```python
from build123d import *

# Parameters (mm, degrees)
SKETCH1_R                = 0.45
BOSS_EXTRUDE1_DEPTH      = 1
SKETCH2_R                = 0.75
BOSS_EXTRUDE2_DEPTH      = 0.5
SKETCH3_R                = 0.125
BOSS_EXTRUDE3_DEPTH      = 4
BOSS_EXTRUDE3_DEPTH_BACK = 20
CHAMFER1_SIZE            = 0.1


with BuildPart() as part:
    # Sketch1 → Boss-Extrude1 (new body)
    with BuildSketch(Plane(origin=(0, 0, 0), x_dir=(1, 0, 0), z_dir=(0, 1, 0))):
        Circle(SKETCH1_R)
    extrude(amount=BOSS_EXTRUDE1_DEPTH)

    # Sketch2 → Boss-Extrude2 (add)
    with BuildSketch(Plane(origin=(0, 1, 0), x_dir=(1, 0, 0), z_dir=(0, 1, 0))):
        Circle(SKETCH2_R)
    extrude(amount=BOSS_EXTRUDE2_DEPTH)

    # Sketch3 → Boss-Extrude3 (add, two sides)
    with BuildSketch(Plane.XY) as boss_extrude3_sk:
        with Locations((0, 1.25)):
            Circle(SKETCH3_R)
    extrude(amount=BOSS_EXTRUDE3_DEPTH)
    extrude(boss_extrude3_sk.sketch, amount=-BOSS_EXTRUDE3_DEPTH_BACK)

    # Chamfer1
    chamfer1_edges = [part.edges().sort_by_distance(p)[0] for p in [
        (-0.75, 1.5, 0),
    ]]
    chamfer(chamfer1_edges, length=CHAMFER1_SIZE)


solid = part.part
```
For this review, take the finished solid that the model builds, in its own axes (mm). A direction names the side the tool comes from. Give positions to 0.01 mm unless a question says otherwise; leave off trailing zeros. Order: outer loops, then holes, each group sorted by start corner. A loop starts at its lowest first (then second) coordinate and runs counter-clockwise, first axis right, second up.
1) Wall thickness on line 1 (Y direction, x = 0, z = -6) (3 decimals); line 2 (Z direction, x = -0.15, y = 0.9); line 3 (Z direction, x = -0.3, y = 0.25): over which ranges is each line inside the solid? List them lowest first.
2) For faces 1 (the face through (0, 1.5, 0)), 2 (the face through (0.429, 0.493, -0.135)), list the 3-axis set-ups (+Z, -Z, +X, -X, +Y, -Y) from which the entire face can be reached by the end or side of a thin tool; tool diameter is ignored.
3) Take a section at A-A (z = 0). Give the boundary of the cut face in (x, y), then the cut area to 3 significant figures.
4) Take a section at B-B (y = 0.45). Give the boundary of the cut face in (x, z), then the cut area to 3 significant figures.
Derived:
1. line 1: y = 1.125 to 1.375
1. line 2: z = -0.42 to 0.42
1. line 3: z = -0.34 to 0.34
2. face 1: +Z, -Z, +X, -X, +Y
2. face 2: -Y
3. outline: (-0.75, 1) - (-0.45, 1) - (-0.45, 0) - (0.45, 0) - (0.45, 1) - (0.75, 1) - (0.75, 1.4) - (0.65, 1.5) - (-0.65, 1.5) - (-0.75, 1.4) - close
3. area: 1.64 mm2
4. outline: circle Ø0.9 at (0, 0)
4. area: 0.636 mm2
